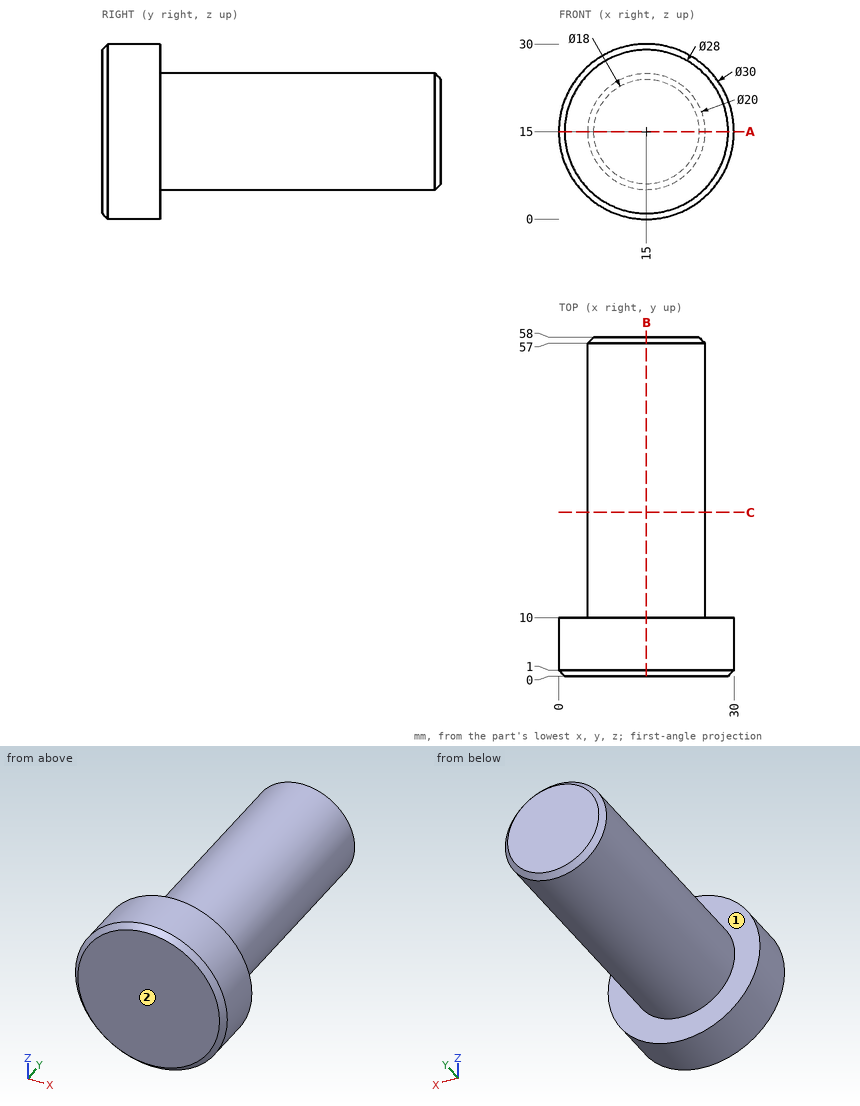
Here's the drawing with two shaded views (mm, measured from the low corner). I have some questions. A direction names the side the tool comes from. Give positions to 0.01 mm unless a question says otherwise; leave off trailing zeros. Loops run counter-clockwise (first coordinate to the right, second up) from the corner with the lowest first, then second, coordinate; pieces in that order, holes last. Notation, with made-up numbers: M 83,-39.75 L 135,-39.75 A21 ccw 135,-6.75 Z; hole C -12.75,33 d4. An arc over 180 degrees is marked long. Answer in a Markdown table with one row per item.
1. For pin 1 Ø6 at (y, z) = (25, 20.5) entering from -X; pin 2 Ø8 at (x, y) = (21.5, 16.5) entering from -Z; pin 3 Ø5 at (y, z) = (12, 8.5) entering from -X, each with a flat end and sliding along its axis, tell me the tip position at first contact or that it passes through.
Taken from the geometry:
| item | result |
|---|---|
| pin 1 | stops at x = 5.32 |
| pin 2 | stops at z = 5.32 |
| pin 3 | stops at x = 0.86 |
2. Suppose I cut it at A-A on z = 15. Write out the boundary of the cut face in (x, y).
Taken from the geometry:
| item | result |
|---|---|
| outline | M 0,1 L 1,0 L 29,0 L 30,1 L 30,10 L 25,10 L 25,57 L 24,58 L 6,58 L 5,57 L 5,10 L 0,10 Z |
3. Which directions (+Z, -Z, +X, -X, +Y, -Y) give clear straight access to the entire face, cutting with the end or side of a thin tool? Please do the marked faces 1 and 2.
Taken from the geometry:
| item | result |
|---|---|
| face 1 | +Y |
| face 2 | +Z, -Z, +X, -X, -Y |
4. Suppose I cut it at C-C on y = 28. Write out the boundary of the cut face in (x, z), plus the area to 3 significant figures.
Taken from the geometry:
| item | result |
|---|---|
| outline | C 15,15 d20 |
| area | 314 mm² |
5. Suppose I cut it at B-B on x = 15. Write out the boundary of the cut face in (y, z), plus the area to 3 significant figures.
Taken from the geometry:
| item | result |
|---|---|
| outline | M 0,1 L 1,0 L 10,0 L 10,5 L 57,5 L 58,6 L 58,24 L 57,25 L 10,25 L 10,30 L 1,30 L 0,29 Z |
| area | 1,260 mm² |
6. If I drill on line 1 along Y through (x, z) = (5, 5.75); line 2 along Z through (x, y) = (15.5, 33); line 3 along X through (y, z) = (38.5, 14.75), over which ranges is the centre line in solid material (lowest first)?
Taken from the geometry:
| item | result |
|---|---|
| line 1 | y = 0 to 10 |
| line 2 | z = 5.01 to 24.99 |
| line 3 | x = 5 to 25 |
